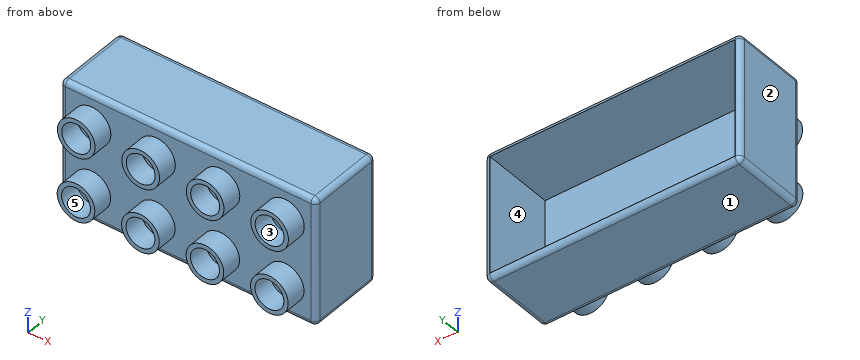
from build123d import *

# Parameters (mm, degrees)
F0_W     = 63.5
F0_H     = 19.05
F1_DEPTH = 31.75
F2_T     = -1.3208
F3_R     = 4.6736
F3_R_2   = 3.5941
F4_DEPTH = 5.08
F5_R     = 1.27


with BuildPart() as f1:
    # F0 (on Top) → F1 (new body)
    with BuildSketch(Plane.XY):
        with Locations((-26.116837, 21.650621)):
            Rectangle(F0_W, F0_H)
    extrude(amount=F1_DEPTH)

    # F2
    f2_openings = [f1.faces().sort_by_distance(p)[0] for p in [
        (-26.116837, 31.175621, 15.875),
    ]]
    offset(amount=F2_T, openings=f2_openings)

    # F3 (on face) → F4 (join)
    with BuildSketch(Plane.XZ.offset(-12.125621)):
        with Locations((-49.992837, 23.876)):
            Circle(F3_R)
        with Locations((-49.992837, 23.876)):
            Circle(F3_R_2, mode=Mode.SUBTRACT)
        with Locations((-33.990837, 23.876)):
            Circle(F3_R)
        with Locations((-33.990837, 23.876)):
            Circle(F3_R_2, mode=Mode.SUBTRACT)
        with Locations((-17.988837, 23.876)):
            Circle(F3_R)
        with Locations((-17.988837, 23.876)):
            Circle(F3_R_2, mode=Mode.SUBTRACT)
        with Locations((-1.986837, 23.876)):
            Circle(F3_R)
        with Locations((-1.986837, 23.876)):
            Circle(F3_R_2, mode=Mode.SUBTRACT)
        with Locations((-50.052113, 7.87411)):
            Circle(F3_R)
        with Locations((-50.052113, 7.87411)):
            Circle(F3_R_2, mode=Mode.SUBTRACT)
        with Locations((-34.050113, 7.87411)):
            Circle(F3_R)
        with Locations((-34.050113, 7.87411)):
            Circle(F3_R_2, mode=Mode.SUBTRACT)
        with Locations((-18.048113, 7.87411)):
            Circle(F3_R)
        with Locations((-18.048113, 7.87411)):
            Circle(F3_R_2, mode=Mode.SUBTRACT)
        with Locations((-2.046113, 7.87411)):
            Circle(F3_R)
        with Locations((-2.046113, 7.87411)):
            Circle(F3_R_2, mode=Mode.SUBTRACT)
    extrude(amount=F4_DEPTH)

    # F5
    f5_edges = [f1.edges().sort_by_distance(p)[0] for p in [
        (-26.116837, 31.175621, 0),
        (-57.866837, 21.650621, 0),
        (-26.116837, 12.125621, 0),
        (5.633163, 21.650621, 0),
        (-57.866837, 31.175621, 15.875),
        (-57.866837, 12.125621, 15.875),
        (-57.866837, 21.650621, 31.75),
        (-26.116837, 31.175621, 31.75),
        (-26.116837, 12.125621, 31.75),
        (5.633163, 21.650621, 31.75),
        (5.633163, 12.125621, 15.875),
        (5.633163, 31.175621, 15.875),
    ]]
    fillet(f5_edges, radius=F5_R)


solid = f1.part
Read the model definition and answer for the solid it produces. Units are mm, in the model's axes. Face numbers are marked on the shaded views. A direction names the side the tool comes from. Coordinates: 2 decimals unless noted, no trailing zeros. Loops run counter-clockwise (first coordinate to the right, second up) from the corner with the lowest first, then second, coordinate; pieces in that order, holes last.
Q1. The part is cut by section B-B on x = -42.5. Write down the section's boundary in (y, z).
Q2. Each of these flat-tipped pins is pushed along its axis until it touches: pin 1 Ø6 at (x, z) = (-34.05, 7.87) entering from +Y; pin 2 Ø2 at (x, z) = (-1.5, 22.5) entering from -Y. Where does it stop, or does it pass through?
Q3. The part is cut by section A-A on y = 27.5. Write down the section's boundary in (x, z), and give its area (3 significant figures).
Q4. The part is cut by section C-C on z = 14. Write down the section's boundary in (x, y), and give its area (3 significant figures).
Q5. The mould has two halves that part along Z. Classify the marked faces 1, 2 and 3: +Z half, -Z half, draft (parallel to the pull), parting line (faces both ways), or undercut.
Q6. Which of the six approach directions +Z, -Z, +X, -X, +Y, -Y give full straight-line access (tool end or side, diameter ignored) to the marked faces 4 and 5?
Q7. The part is cut by section D-D on x = -51.5. Write down the section's boundary in (y, z), and give its area (3 significant figures).
Q8. Consider probe 1 along Z at (x, y) = (-49, 17.5); probe 2 along X at (y, z) = (28, 29.5); probe 3 along Y at (x, z) = (-18, 9). Determine where each line is inside the solid, lowest interval first.
Results below:
1. outline: (12.13, 1.27) arc R1.27 ccw to (13.4, 0) - (29.91, 0) arc R1.27 ccw to (31.18, 1.27) - (31.18, 1.32) - (13.45, 1.32) - (13.45, 30.43) - (31.18, 30.43) - (31.18, 30.48) arc R1.27 ccw to (29.91, 31.75) - (13.4, 31.75) arc R1.27 ccw to (12.13, 30.48) - close
2. pin 1: stops at y = 13.45
2. pin 2: stops at y = 12.13
3. outline: (-57.87, 1.27) arc R1.27 ccw to (-56.6, 0) - (4.36, 0) arc R1.27 ccw to (5.63, 1.27) - (5.63, 30.48) arc R1.27 ccw to (4.36, 31.75) - (-56.6, 31.75) arc R1.27 ccw to (-57.87, 30.48) - close; hole (-56.55, 1.32) - (4.31, 1.32) - (4.31, 30.43) - (-56.55, 30.43) - close
3. area: 243 mm2
4. outline: (-57.87, 13.4) arc R1.27 ccw to (-56.6, 12.13) - (4.36, 12.13) arc R1.27 ccw to (5.63, 13.4) - (5.63, 29.91) arc R1.27 ccw to (4.36, 31.18) - (4.31, 31.18) - (4.31, 13.45) - (-56.55, 13.45) - (-56.55, 31.18) - (-56.6, 31.18) arc R1.27 ccw to (-57.87, 29.91) - close
4. area: 129 mm2
5. face 1: -Z half
5. face 2: draft
5. face 3: undercut
6. face 4: +Y
6. face 5: -Y
7. outline: (7.05, 3.43) - (12.13, 3.43) - (12.13, 1.27) arc R1.27 ccw to (13.4, 0) - (29.91, 0) arc R1.27 ccw to (31.18, 1.27) - (31.18, 1.32) - (13.45, 1.32) - (13.45, 30.43) - (31.18, 30.43) - (31.18, 30.48) arc R1.27 ccw to (29.91, 31.75) - (13.4, 31.75) arc R1.27 ccw to (12.13, 30.48) - (12.13, 28.3) - (7.05, 28.3) - (7.05, 27.14) - (12.13, 27.14) - (12.13, 20.61) - (7.05, 20.61) - (7.05, 19.45) - (12.13, 19.45) - (12.13, 12.32) - (7.05, 12.32) - (7.05, 11.16) - (12.13, 11.16) - (12.13, 4.58) - (7.05, 4.58) - close
7. area: 111 mm2
8. probe 1: z = 0 to 1.32, 30.43 to 31.75
8. probe 2: x = -57.87 to -56.55, 4.31 to 5.63
8. probe 3: y = 12.13 to 13.45
